For this review, take the finished solid that the model builds, in its own axes (mm). A direction names the side the tool comes from. Give positions to 0.01 mm unless a question says otherwise; leave off trailing zeros. Order: outer loops, then holes, each group sorted by start corner. A loop starts at its lowest first (then second) coordinate and runs counter-clockwise, first axis right, second up. Notation, with made-up numbers: (0, 87) - (43, 87) arc R30 cw to (43, 112) - close; hole circle Ø5 at (-31, 24). An arc over 180 degrees is marked (long way). Answer as a JSON object with one key per item and string values. Group by question number.
from build123d import *

# Parameters (mm, degrees)
SKETCH1_W           = 12.7
SKETCH1_H           = 5.842
BOSS_EXTRUDE1_DEPTH = 5.842
FILLET1_R           = 1.5875
CUT_EXTRUDE1_DEPTH  = 96.902317244
SKETCH3_R           = 3.175
CUT_EXTRUDE2_DEPTH  = 96.902317244
SKETCH4_R           = 3.175
BOSS_EXTRUDE2_DEPTH = 5.842
FILLET2_R           = 3.175


with BuildPart() as part:
    # Sketch1 → Boss-Extrude1 (new body)
    with BuildSketch(Plane(origin=(0, 0, 0), x_dir=(1, 0, 0), z_dir=(0, 1, 0))):
        Polygon((19.05, -21.1058), (25.5, -21.1058), (25.5, 21.1058), (19.05, 21.1058), (19.05, 26.9478), (25.5, 26.9478), (25.5, 30.1228), (-25.5, 30.1228), (-25.5, 26.9478), (-19.05, 26.9478), (-19.05, 21.1058), (-25.5, 21.1058), (-25.5, -21.1058), (-19.05, -21.1058), (-19.05, -26.9478), (-25.5, -26.9478), (-31.342, -26.9478), (-31.342, -39.6478), (-25.5, -39.6478), (-25.5, -65.0478), (-31.342, -65.0478), (-31.342, -77.7478), (-25.5, -77.7478), (-25.5, -90.4478), (-6.35, -90.4478), (-6.35, -84.0978), (6.35, -84.0978), (6.35, -90.4478), (25.5, -90.4478), (25.5, -77.7478), (31.342, -77.7478), (31.342, -65.0478), (25.5, -65.0478), (25.5, -39.6478), (31.342, -39.6478), (31.342, -26.9478), (25.5, -26.9478), (19.05, -26.9478), align=None)
        with Locations((0, -24.0268)):
            Rectangle(SKETCH1_W, SKETCH1_H, mode=Mode.SUBTRACT)
        with Locations((0, 24.0268)):
            Rectangle(SKETCH1_W, SKETCH1_H, mode=Mode.SUBTRACT)
    extrude(amount=BOSS_EXTRUDE1_DEPTH)

    # Fillet1
    fillet1_edges = [part.edges().sort_by_distance(p)[0] for p in [
        (-25.5, 2.921, -30.1228),
        (25.5, 2.921, -30.1228),
    ]]
    fillet(fillet1_edges, radius=FILLET1_R)

    # Sketch2 → Cut-Extrude1 (cut, through all)
    with BuildSketch(Plane(origin=(0, 5.842, 0), x_dir=(1, 0, 0), z_dir=(0, 1, 0))):
        Polygon((-19.15, -44.2198), (-19.15, -42.9498), (-15.975, -42.9498), (-15.975, -44.2198), (-12.292, -44.2198), (-12.292, -47.7758), (-15.975, -47.7758), (-15.975, -49.0458), (-19.15, -49.0458), (-19.15, -47.7758), (-25.5, -47.7758), (-25.5, -44.2198), align=None)
        Polygon((12.292, -44.2198), (15.975, -44.2198), (15.975, -42.9498), (19.15, -42.9498), (19.15, -44.2198), (25.5, -44.2198), (25.5, -47.7758), (19.15, -47.7758), (19.15, -49.0458), (15.975, -49.0458), (15.975, -47.7758), (12.292, -47.7758), align=None)
        Polygon((19.15, -85.8758), (19.15, -87.1458), (15.975, -87.1458), (15.975, -85.8758), (12.292, -85.8758), (12.292, -82.3198), (15.975, -82.3198), (15.975, -81.0498), (19.15, -81.0498), (19.15, -82.3198), (25.5, -82.3198), (25.5, -85.8758), align=None)
        Polygon((-12.292, -85.8758), (-15.975, -85.8758), (-15.975, -87.1458), (-19.15, -87.1458), (-19.15, -85.8758), (-25.5, -85.8758), (-25.5, -82.3198), (-19.15, -82.3198), (-19.15, -81.0498), (-15.975, -81.0498), (-15.975, -82.3198), (-12.292, -82.3198), align=None)
    extrude(amount=-CUT_EXTRUDE1_DEPTH, mode=Mode.SUBTRACT)

    # Sketch3 → Cut-Extrude2 (cut, through all)
    with BuildSketch(Plane(origin=(0, 5.842, 0), x_dir=(1, 0, 0), z_dir=(0, 1, 0))):
        with Locations(Location((0, 0, 0), (0, 0, 270))):
            Circle(SKETCH3_R)
        with Locations(Location((-12.7, -65.0478, 0), (0, 0, 270))):
            Circle(SKETCH3_R)
        with Locations(Location((12.7, -65.0478, 0), (0, 0, 90))):
            Circle(SKETCH3_R)
        with Locations(Location((0, -39.6478, 0), (0, 0, 270))):
            Circle(SKETCH3_R)
    extrude(amount=-CUT_EXTRUDE2_DEPTH, mode=Mode.SUBTRACT)

    # Sketch4 → Boss-Extrude2 (add)
    with BuildSketch(Plane(origin=(0, 5.842, 0), x_dir=(1, 0, 0), z_dir=(0, 1, 0))):
        with BuildLine():
            Line((-19.05, 30.1228), (-4.403989261, 44.222445188))
            ThreePointArc((-4.403989261, 44.222445188), (0, 45.9978), (4.403989261, 44.222445188))
            Line((4.403989261, 44.222445188), (19.05, 30.1228))
            Line((19.05, 30.1228), (-19.05, 30.1228))
        make_face()
        with Locations(Location((0, 39.6478, 0), (0, 0, 270))):
            Circle(SKETCH4_R, mode=Mode.SUBTRACT)
    extrude(amount=-BOSS_EXTRUDE2_DEPTH)

    # Fillet2
    fillet2_edges = [part.edges().sort_by_distance(p)[0] for p in [
        (-19.05, 2.921, -30.1228),
        (19.05, 2.921, -30.1228),
    ]]
    fillet(fillet2_edges, radius=FILLET2_R)


solid = part.part
1) Consider section B-B (z = 0). Give the boundary of the cut face in (x, y) (3 decimals).
2) For faces 5 (the face through (-28, 3, 77.748)), 6 (the face through (25.5, 3, 0)), 7 (the face through (19.05, 3, -24)), 8 (the face through (-25.5, 3, 0)), 9 (the face through (-22, 3, 44.22)), list the 3-axis set-ups (+Z, -Z, +X, -X, +Y, -Y) from which the entire face can be reached by the end or side of a thin tool; tool diameter is ignored.
3) Consider section C-C (x = -1.5). Give the boundary of the cut face in (y, z), plus the area to 3 significant figures.
4) Mouldability with a two-part tool opening along Z and no side actions: class faces 1 (the face through (6.35, 3, 87)), 2 (the face through (-22, 3, -30.123)), 3 (the face through (25.5, 3, 42)), 4 (the face through (25.5, 3, 57)) as released by +Z, released by -Z, zero draft, split by the parting line, or undercut.
5) Consider section D-D (y = 4.95). Give the number of separate pieces and of enclosed holes in the cut face, plus the area to 3 significant figures.
6) For line 1 (Z direction, x = -18, y = 0.75); line 2 (Z direction, x = -18.5, y = 3.1); line 3 (X direction, y = 1.6, z = 64), list the stretches that pass through material, from the lowest coordinate up.
7) For pin 1 (1 mm diameter, centred on y = 3, z = 86.5, fed in from +X); pin 2 (1.8 mm diameter, centred on y = 2.5, z = 58.5, fed in from -X); pin 3 (3 mm diameter, centred on x = 28.5, y = 4, fed in from +Z); pin 4 (5.5 mm diameter, centred on x = -12.7, z = 65.05, fed in from -Y), all flat-tipped, find the tip position at first contact; note any pin that passes through.
8) Consider section A-A (x = 22). Give the boundary of the cut face in (y, z).
Result set:
{
 "1": {"outline": "(-25.5, 0) - (-3.175, 0) - (-3.175, 5.842) - (-25.5, 5.842) - close; (3.175, 0) - (25.5, 0) - (25.5, 5.842) - (3.175, 5.842) - close"},
 "2": {"face 5": "+Z, -X, +Y, -Y", "face 6": "-Z, +X, +Y, -Y", "face 7": "+X, +Y, -Y", "face 8": "-Z, -X, +Y, -Y", "face 9": "-X, +Y, -Y"},
 "3": {"outline": "(0, -45.82) - (5.84, -45.82) - (5.84, -42.45) - (0, -42.45) - close; (0, -36.85) - (5.84, -36.85) - (5.84, -26.95) - (0, -26.95) - close; (0, -21.11) - (5.84, -21.11) - (5.84, -2.8) - (0, -2.8) - close; (0, 2.8) - (5.84, 2.8) - (5.84, 21.11) - (0, 21.11) - close; (0, 26.95) - (5.84, 26.95) - (5.84, 36.85) - (0, 36.85) - close; (0, 42.45) - (5.84, 42.45) - (5.84, 84.1) - (0, 84.1) - close", "area": "593 mm2"},
 "4": {"face 1": "zero draft", "face 2": "released by -Z", "face 3": "undercut", "face 4": "undercut"},
 "5": {"separate pieces": "1", "enclosed holes": "7", "area": "6,030 mm2"},
 "6": {"line 1": "z = -31.13 to 42.95, 49.05 to 81.05, 87.15 to 90.45", "line 2": "z = -30.7 to 42.95, 49.05 to 81.05, 87.15 to 90.45", "line 3": "x = -25.5 to -15.7, -9.7 to 9.7, 15.7 to 25.5"},
 "7": {"pin 1": "stops at x = 25.5", "pin 2": "stops at x = -25.5", "pin 3": "stops at z = 77.75", "pin 4": "passes through"},
 "8": {"outline": "(0, -30.12) - (5.84, -30.12) - (5.84, -26.95) - (0, -26.95) - close; (0, -21.11) - (5.84, -21.11) - (5.84, 21.11) - (0, 21.11) - close; (0, 26.95) - (5.84, 26.95) - (5.84, 44.22) - (0, 44.22) - close; (0, 47.78) - (5.84, 47.78) - (5.84, 82.32) - (0, 82.32) - close; (0, 85.88) - (5.84, 85.88) - (5.84, 90.45) - (0, 90.45) - close"}
}
